```python
from build123d import *

# Parameters (mm, degrees)
SKETCH_1_R          = 1.5
EXTRUDE_1_DEPTH     = 10.9
SKETCH_2_R          = 1.3
CUT_EXTRUDE_1_DEPTH = 13
SKETCH_5_R          = 5.1
CUT_EXTRUDE_3_DEPTH = 37.903132997
SKETCH_6_R          = 1.5
CUT_EXTRUDE_4_DEPTH = 37.903132997
SKETCH_7_W          = 28.07
SKETCH_7_H          = 25
CUT_EXTRUDE_5_DEPTH = 37.903132997
FILLET_2_R          = 3


with BuildPart() as part:
    # ｽｹｯﾁ1 → ﾎﾞｽ - 押し出し1 (new body)
    with BuildSketch(Plane.XY):
        Polygon((9.035, 12.6), (9.035, 20), (-29.035, 20), (-29.035, -20), (9.035, -20), (9.035, 2.5), (16.035, 2.5), (16.035, -20), (29.035, -20), (29.035, 20), (16.035, 20), (16.035, 12.6), align=None)
        with Locations((4.035, -2.45)):
            Circle(SKETCH_1_R, mode=Mode.SUBTRACT)
        with Locations((22.535, -2.45)):
            Circle(SKETCH_1_R, mode=Mode.SUBTRACT)
        with Locations((4.035, 7.55)):
            Circle(SKETCH_1_R, mode=Mode.SUBTRACT)
        with Locations((22.535, 7.55)):
            Circle(SKETCH_1_R, mode=Mode.SUBTRACT)
        with Locations((4.035, 15.05)):
            Circle(SKETCH_1_R, mode=Mode.SUBTRACT)
    extrude(amount=EXTRUDE_1_DEPTH)

    # ｽｹｯﾁ2 → ｶｯﾄ - 押し出し1 (cut)
    with BuildSketch(Plane(origin=(29.035, 0, 0), x_dir=(0, 0, -1), z_dir=(1, 0, 0))):
        with Locations((-5.45, 17)):
            Circle(SKETCH_2_R)
        with Locations(Location((-5.45, -17, 0), (0, 0, 270))):
            Circle(SKETCH_2_R)
    extrude(amount=-CUT_EXTRUDE_1_DEPTH, mode=Mode.SUBTRACT)

    # ｽｹｯﾁ5 → ｶｯﾄ - 押し出し3 (cut, through all)
    with BuildSketch(Plane.XY.offset(10.9)):
        with Locations((-29.035, 24)):
            Circle(SKETCH_5_R)
        with Locations((-8.935, 24)):
            Circle(SKETCH_5_R)
    extrude(amount=-CUT_EXTRUDE_3_DEPTH, mode=Mode.SUBTRACT)

    # ｽｹｯﾁ6 → ｶｯﾄ - 押し出し4 (cut, through all)
    with BuildSketch(Plane.XY.offset(10.9)):
        with Locations((-24.235, -15)):
            Circle(SKETCH_6_R)
        with Locations((-14.235, -15)):
            Circle(SKETCH_6_R)
    extrude(amount=-CUT_EXTRUDE_4_DEPTH, mode=Mode.SUBTRACT)

    # ｽｹｯﾁ7 → ｶｯﾄ - 押し出し5 (cut, through all)
    with BuildSketch(Plane.XY.offset(10.9)):
        with Locations((-15, 7.5)):
            Rectangle(SKETCH_7_W, SKETCH_7_H)
    extrude(amount=-CUT_EXTRUDE_5_DEPTH, mode=Mode.SUBTRACT)

    # ﾌｨﾚｯﾄ2
    # the kernel refuses this fillet: 3 mm, written as the material it adds along each edge
    with BuildSketch(Plane(origin=(-0.965, -5, 10.9), x_dir=(-1, 0, 0), z_dir=(0, 0, -1))) as fillet_2_piece_1:
        with BuildLine():
            CenterArc((FILLET_2_R, FILLET_2_R), FILLET_2_R, 180, 90)
            Line((0, FILLET_2_R), (0, 0))
            Line((0, 0), (FILLET_2_R, 0))
        make_face()
    extrude(amount=10.9)
    # the kernel refuses this fillet: 3 mm, written as the material it takes off along each edge
    with BuildSketch(Plane(origin=(-29.035, -5, 18.4), x_dir=(0, -1, 0), z_dir=(0, 0, -1)), Plane(origin=(-0.965, 20, 18.4), x_dir=(0, -1, 0), z_dir=(0, 0, -1))) as fillet_2_2_piece_1:
        with BuildLine():
            CenterArc((FILLET_2_R, -FILLET_2_R), FILLET_2_R, 90, 90)
            Line((0, -FILLET_2_R), (0, 0))
            Line((0, 0), (FILLET_2_R, 0))
        make_face()
    extrude(amount=25.9, mode=Mode.SUBTRACT)
    with BuildSketch(Plane(origin=(9.035, -20, -7.5), x_dir=(0, 1, 0), z_dir=(0, 0, 1)), Plane(origin=(-29.035, -20, -7.5), x_dir=(1, 0, 0), z_dir=(0, 0, 1)), Plane(origin=(9.035, 20, -7.5), x_dir=(-1, 0, 0), z_dir=(0, 0, 1)), Plane(origin=(16.035, 20, -7.5), x_dir=(0, -1, 0), z_dir=(0, 0, 1)), Plane(origin=(16.035, -20, -7.5), x_dir=(1, 0, 0), z_dir=(0, 0, 1))) as fillet_2_2_piece_2:
        with BuildLine():
            CenterArc((FILLET_2_R, FILLET_2_R), FILLET_2_R, 180, 90)
            Line((0, FILLET_2_R), (0, 0))
            Line((0, 0), (FILLET_2_R, 0))
        make_face()
    extrude(amount=25.9, mode=Mode.SUBTRACT)


solid = part.part
```
CAD build for the part. Positions are in the model's coordinates, mm. A direction names the side the tool comes from. Round coordinates to 2 decimals unless told otherwise and drop trailing zeros. Order: outer loops, then holes, each group sorted by start corner. A loop starts at its lowest first (then second) coordinate and runs counter-clockwise, first axis right, second up.
Item 1: Saw through at B-B on z = 8.25. State how many separate pieces and enclosed holes the cut face has, then the cut area to 3 significant figures.
Item 2: Saw through at D-D on y = 15.05. Write the cut outline in (x, z) (3 decimals), then the cut area to 3 significant figures.
Item 3: Saw through at A-A on y = -15. Write the cut outline in (x, z) (3 decimals), then the cut area to 3 significant figures.
Item 4: Probe line 1 along X through (y, z) = (-12, 4) (3 decimals); line 2 along X through (y, z) = (2, 8) (3 decimals); line 3 along Y through (x, z) = (16, 9.25). List the from-to ranges inside material, lowest first.
Item 5: Tool access for faces 4 (the face through (-15, -5, 6)), 5 (the face through (16.937, 19.145, 5.374)), 6 (the face through (12, 2.5, 5)): list every direction of +Z, -Z, +X, -X, +Y, -Y with a clear straight run to the whole face (end or side of a thin tool).
Item 6: Saw through at C-C on x = -25. Write the cut outline in (y, z).
Item 7: Mould opens along X. For faces 1 (the face through (24, 20, 5)), 2 (the face through (9.035, -7, 5)), 3 (the face through (-0.11, 19.1, 5.53)) say: pulls with the +X half, pulls with the -X half, needs draft (parallel to the pull), parting line crosses it, or undercut.
Item 8: Pin check, flat tips, straight feed: pin 1 (2.5 mm diameter, centred on y = 17, z = 5.45, fed in from -X) (3 decimals); pin 2 (6 mm diameter, centred on x = -3.5, z = 9, fed in from +Y); pin 3 (2 mm diameter, centred on x = 14, z = 8, fed in from +Y). Stop position of each tip, or through.
Reported:
1. separate pieces: 1
1. enclosed holes: 7
1. area: 1,350 mm2
2. outline: (-0.965, 0) - (2.535, 0) - (2.535, 10.9) - (-0.965, 10.9) - close; (5.535, 0) - (9.035, 0) - (9.035, 10.9) - (5.535, 10.9) - close; (16.035, 0) - (29.035, 0) - (29.035, 10.9) - (16.035, 10.9) - close
2. area: 218 mm2
3. outline: (-29.035, 0) - (-25.735, 0) - (-25.735, 10.9) - (-29.035, 10.9) - close; (-22.735, 0) - (-15.735, 0) - (-15.735, 10.9) - (-22.735, 10.9) - close; (-12.735, 0) - (9.035, 0) - (9.035, 10.9) - (-12.735, 10.9) - close; (16.035, 0) - (29.035, 0) - (29.035, 10.9) - (16.035, 10.9) - close
3. area: 491 mm2
4. line 1: x = -29.035 to 9.035, 16.035 to 29.035
4. line 2: x = -0.965 to 9.035, 16.035 to 29.035
4. line 3: y = 2.5 to 12.6
5. face 4: +Z, -Z, -X, +Y
5. face 5: +Z, -Z, +Y
5. face 6: +Z, -Z, -Y
6. outline: (-20, 0) - (-16.29, 0) - (-16.29, 10.9) - (-20, 10.9) - close; (-13.71, 0) - (-5, 0) - (-5, 10.9) - (-13.71, 10.9) - close
7. face 1: needs draft
7. face 2: undercut
7. face 3: pulls with the -X half
8. pin 1: stops at x = -0.965
8. pin 2: stops at y = 18.6
8. pin 3: stops at y = 12.6
